For this review, take the finished solid that the model builds, in its own axes (mm). Round coordinates to 2 decimals unless told otherwise and drop trailing zeros. Order: outer loops, then holes, each group sorted by start corner. A loop starts at its lowest first (then second) coordinate and runs counter-clockwise, first axis right, second up. Notation, with made-up numbers: (-23.5, 41) -> (-15.5, 41) arc R17 ccw to (-15.5, 64) -> close; hole circle Ø7 at (30.5, 27). An arc over 180 degrees is marked (long way). Use a Markdown table: item, result. Add a question column.
1) Consider section B-B (x = -0.5). State the section outline as (y, z) points, plus the area to 3 significant figures.
2) Consider section C-C (z = -0.65). State the section outline as (x, y) points.
3) Wall thickness on line 1 along X through (y, z) = (7, 0); line 2 along Y through (x, z) = (-2, -0.7); line 3 along Z through (x, y) = (1.5, -1): over which ranges is each line inside the solid? List them lowest first. Write a range as [from, to].
4) Consider section A-A (y = 3). State the section outline as (x, z) points.
5) Clearance check with a flat-ended pin moving along its axis: P1, Ø1.2, axis at x = 0, z = -0.5, coming from the -Y side. State where the tip first meets the part, or that it passes through.
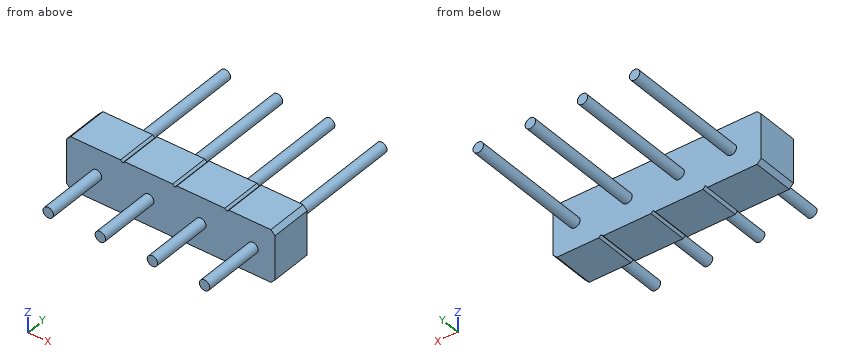
```python
from build123d import *

# Parameters (mm, degrees)
IZIM1_R                          = 0.25
Y_KSEKLIK_EKSTR_ZYON1_DEPTH      = 2
IZIM2_R                          = 0.25
Y_KSEKLIK_EKSTR_ZYON2_DEPTH      = 6
Y_KSEKLIK_EKSTR_ZYON2_DEPTH_BACK = 5


with BuildPart() as part:
    # Çizim1 → Yükseklik-Ekstrüzyon1 (new body)
    with BuildSketch(Plane(origin=(0, 0, 0), x_dir=(1, 0, 0), z_dir=(0, 1, 0))):
        Polygon((-4.8, 1.25), (-2.412060191, 1.25), (-2.311389974, 1.122349253), (-2.210719757, 1.25), (0.088610026, 1.25), (0.188610026, 1.15), (0.288610026, 1.25), (2.588610026, 1.25), (2.688610026, 1.15), (2.788610026, 1.25), (4.8, 1.25), (5, 1.05), (5, -1.05), (4.8, -1.25), (2.788610026, -1.25), (2.688610026, -1.15), (2.588610026, -1.25), (0.288610026, -1.25), (0.188610026, -1.15), (0.088610026, -1.25), (-2.211389974, -1.25), (-2.311389974, -1.15), (-2.411389974, -1.25), (-4.8, -1.25), (-5, -1.05), (-5, 1.05), align=None)
        with Locations((-3.561389974, 0)):
            Circle(IZIM1_R, mode=Mode.SUBTRACT)
        with Locations((-1.061389974, 0)):
            Circle(IZIM1_R, mode=Mode.SUBTRACT)
        with Locations((1.438610026, 0)):
            Circle(IZIM1_R, mode=Mode.SUBTRACT)
        with Locations((3.938610026, 0)):
            Circle(IZIM1_R, mode=Mode.SUBTRACT)
    extrude(amount=Y_KSEKLIK_EKSTR_ZYON1_DEPTH)

    # Çizim2 → Yükseklik-Ekstrüzyon2 (add, two sides)
    with BuildSketch(Plane(origin=(0, 2, 0), x_dir=(1, 0, 0), z_dir=(0, 1, 0))) as y_kseklik_ekstr_zyon2_sk:
        with Locations((-3.561389974, 0)):
            Circle(IZIM2_R)
        with Locations((-1.061389974, 0)):
            Circle(IZIM2_R)
        with Locations((1.438610026, 0)):
            Circle(IZIM2_R)
        with Locations((3.938610026, 0)):
            Circle(IZIM2_R)
    extrude(amount=Y_KSEKLIK_EKSTR_ZYON2_DEPTH)
    extrude(y_kseklik_ekstr_zyon2_sk.sketch, amount=-Y_KSEKLIK_EKSTR_ZYON2_DEPTH_BACK)


solid = part.part
```
Results list:
| question | item | result |
|---|---|---|
| 1 | outline | (0, -1.25) -> (2, -1.25) -> (2, 1.25) -> (0, 1.25) -> close |
| 1 | area | 5.00 mm2 |
| 2 | outline | (-5, 0) -> (5, 0) -> (5, 2) -> (-5, 2) -> close |
| 3 | line 1 | [-3.81, -3.31], [-1.31, -0.81], [1.19, 1.69], [3.69, 4.19] |
| 3 | line 2 | [0, 2] |
| 3 | line 3 | [-0.24, 0.24] |
| 4 | outline | circle Ø0.5 at (-3.56, 0); circle Ø0.5 at (-1.06, 0); circle Ø0.5 at (1.44, 0); circle Ø0.5 at (3.94, 0) |
| 5 | P1 | y = 0 |
